Input: part model. Units: mm. Frame: model coordinates. Face numbers are marked on the shaded views. A direction names the side the tool comes from. Coordinates: 2 decimals unless noted, no trailing zeros. Order: outer loops, then holes, each group sorted by start corner. A loop starts at its lowest first (then second) coordinate and runs counter-clockwise, first axis right, second up. Notation, with made-up numbers: (64.5, -9.5) -> (94.5, -9.5) arc R20 cw to (94.5, 14.5) -> close; hole circle Ø3 at (75.25, 39.25). An arc over 180 degrees is marked (long way). Write each question's results on one line, items separated by ' | '.
```python
from build123d import *

# Parameters (mm, degrees)
SKETCH1_W           = 24
SKETCH1_H           = 32
BOSS_EXTRUDE1_DEPTH = 3
SKETCH2_W           = 1.5
SKETCH2_H           = 3
BOSS_EXTRUDE3_DEPTH = 3
SKETCH3_W           = 20
SKETCH3_H           = 5
BOSS_EXTRUDE4_DEPTH = 7


with BuildPart() as part:
    # Sketch1 → Boss-Extrude1 (new body)
    with BuildSketch(Plane(origin=(0, 0, 0), x_dir=(1, 0, 0), z_dir=(0, 1, 0))):
        with Locations((-10.330434783, 1.634782609)):
            Rectangle(SKETCH1_W, SKETCH1_H)
    extrude(amount=BOSS_EXTRUDE1_DEPTH)

    # Sketch2 → Boss-Extrude3 (add)
    with BuildSketch(Plane(origin=(0, 3, 0), x_dir=(1, 0, 0), z_dir=(0, 1, 0))):
        with Locations((-14.580434783, 11.134782609)):
            Rectangle(SKETCH2_W, SKETCH2_H)
        with Locations((-6.080434783, 11.134782609)):
            Rectangle(SKETCH2_W, SKETCH2_H)
    extrude(amount=BOSS_EXTRUDE3_DEPTH)

    # Sketch3 → Boss-Extrude4 (add)
    with BuildSketch(Plane(origin=(0, 6, 0), x_dir=(1, 0, 0), z_dir=(0, 1, 0))):
        with Locations((-10.330434783, 11.134782609)):
            Rectangle(SKETCH3_W, SKETCH3_H)
    extrude(amount=BOSS_EXTRUDE4_DEPTH)


solid = part.part
```
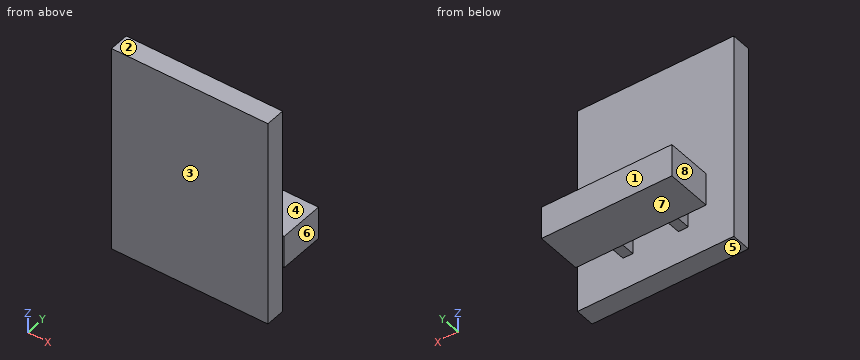
(1) Line query: line 1 along Z through (x, y) = (-10.25, 6.5); line 2 along Y through (x, z) = (-9, -1.5). Output: solid intervals per line, ascending. Write a range as from..to.
Return value:
line 1: -13.63..-8.63 | line 2: 0..3
(2) Cut plane A-A, the plane x = -3.5. Return loops of the section in (y, z), plus the area to 3 significant figures.
Return value:
outline: (0, -17.63) -> (3, -17.63) -> (3, 14.37) -> (0, 14.37) -> close; (6, -13.63) -> (13, -13.63) -> (13, -8.63) -> (6, -8.63) -> close | area: 131 mm2
(3) Reachability of the marked faces 4, 5, 6, 7 and 8 from +Z, -Z, +X, -X, +Y, -Y: full face, straight path, thin tool, end or side. Return the list, or none.
Return value:
face 4: +Z, +X, -X, +Y | face 5: -Z, +X, -X, +Y, -Y | face 6: +Z, -Z, +X, +Y | face 7: -Z, +X, -X, +Y | face 8: +Z, -Z, -X, +Y
(4) Cut plane D-D, the plane z = 3.5. Return loops of the section in (x, y).
Return value:
outline: (-22.33, 0) -> (1.67, 0) -> (1.67, 3) -> (-22.33, 3) -> close
(5) Pin query (flat end, axial travel): P1, Ø12, axis at x = -7, z = 4.5, coming from the +Y side; P2, Ø1.6, axis at x = -6.5, y = 4.5, coming from the -Z side; P3, Ø5.5, axis at y = 9.5, z = -12, coming from the -X side; P4, Ø6, axis at y = 8.5, z = 6, coming from the -X side. Return the tip coordinate at first contact, or that it passes through.
Return value:
P1: y = 3 | P2: z = -12.63 | P3: x = -20.33 | P4: through
(6) Mould query, pull axis Y, two halves, no side actions, for the marked faces 1, 2 and 3. Classes: +Y half, -Y half, draft (parallel to the pull), parting line (faces both ways), or undercut.
Return value:
face 1: +Y half | face 2: draft | face 3: -Y half
(7) Cut plane C-C, the plane y = 12. Return loops of the section in (x, z).
Return value:
outline: (-20.33, -13.63) -> (-0.33, -13.63) -> (-0.33, -8.63) -> (-20.33, -8.63) -> close
(8) Cut plane B-B, the plane z = -10. Return loops of the section in (x, y), plus the area to 3 significant figures.
Return value:
outline: (-22.33, 0) -> (1.67, 0) -> (1.67, 3) -> (-5.33, 3) -> (-5.33, 6) -> (-0.33, 6) -> (-0.33, 13) -> (-20.33, 13) -> (-20.33, 6) -> (-15.33, 6) -> (-15.33, 3) -> (-22.33, 3) -> close; hole (-13.83, 3) -> (-6.83, 3) -> (-6.83, 6) -> (-13.83, 6) -> close | area: 221 mm2
